Design review of the part built by this model. Coordinates are the model's own, in mm. Face numbers are marked on the shaded views. A direction names the side the tool comes from. Coordinates: 2 decimals unless noted, no trailing zeros. Write each loop counter-clockwise with the first axis right and the second up, starting at its lowest first coordinate (ties: lowest second). Pieces come first, ordered by that corner, then holes. Notation, with made-up numbers: (1, 81) -> (5, 81) arc R18 cw to (5, 94) -> close; hole circle Ø3 at (31.5, 79.25). An arc over 180 degrees is marked (long way). One line per question, with ' | ' between items. Start each with the question number.
Q1. Wall thickness on probe 1 along Y at (x, z) = (0, 8.25); probe 2 along Z at (x, y) = (13.5, 1.25); probe 3 along Z at (x, y) = (3, -7.5): over which ranges is each line inside the solid? List them lowest first.
Q2. Add section D-D on z = 8.75. State the section outline as (x, y) points, and give its area (3 significant figures).
Q3. Add section B-B on z = 0.5. State the section outline as (x, y) points, and give its area (3 significant figures).
Q4. Add section A-A on y = 0. State the section outline as (x, z) points.
Q5. Add section C-C on x = -19.5. State the section outline as (y, z) points, and give its area (3 significant figures).
Q6. For the marked faces 1 and 2, list the 3-axis set-ups (+Z, -Z, +X, -X, +Y, -Y) from which the entire face can be reached by the end or side of a thin tool; tool diameter is ignored.
Q7. For P1, Ø1, axis at x = 14, y = 5.5, coming from the +Z side; P2, Ø4, axis at x = -18.5, y = 0, coming from the +Z side; P3, Ø4, axis at x = 7, y = -4.5, coming from the +Z side; P4, Ø2, axis at y = -8, z = 6.5, coming from the +X side, all flat-tipped, find the tip position at first contact; note any pin that passes through.
Q8. Draft analysis for pull direction X (two halves, no side actions). For the marked faces 3, 4 and 5, state which applies: pulls with the +X half, pulls with the -X half, needs draft (parallel to the pull), parting line crosses it, or undercut.
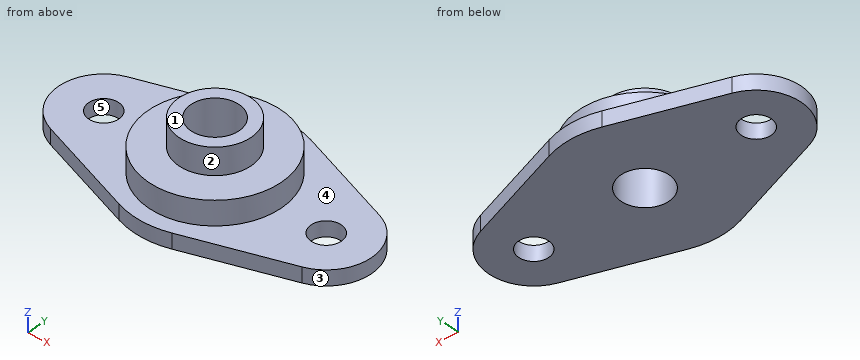
from build123d import *

# Parameters (mm, degrees)
SKETCH2_R           = 4
SKETCH2_R_2         = 2.5
BOSS_EXTRUDE1_DEPTH = 2.5
SKETCH3_R           = 6
SKETCH3_R_2         = 4
BOSS_EXTRUDE2_DEPTH = 10.922
SKETCH4_R           = 11
SKETCH4_R_2         = 6
BOSS_EXTRUDE3_DEPTH = 4


with BuildPart() as part:
    # Sketch2 → Boss-Extrude1 (new body)
    with BuildSketch(Plane.XY):
        with BuildLine():
            ThreePointArc((20.932432432, -7.094594595), (26, 0), (20.932432432, 7.094594595))
            Line((20.932432432, 7.094594595), (4.378378378, 12.77027027))
            ThreePointArc((4.378378378, 12.77027027), (0, 13.5), (-4.378378378, 12.77027027))
            Line((-4.378378378, 12.77027027), (-20.932432432, 7.094594595))
            ThreePointArc((-20.932432432, 7.094594595), (-26, 0), (-20.932432432, -7.094594595))
            Line((-20.932432432, -7.094594595), (-4.378378378, -12.77027027))
            ThreePointArc((-4.378378378, -12.77027027), (0, -13.5), (4.378378378, -12.77027027))
            Line((4.378378378, -12.77027027), (20.932432432, -7.094594595))
        make_face()
        Circle(SKETCH2_R, mode=Mode.SUBTRACT)
        with Locations((18.5, 0)):
            Circle(SKETCH2_R_2, mode=Mode.SUBTRACT)
        with Locations((-18.5, 0)):
            Circle(SKETCH2_R_2, mode=Mode.SUBTRACT)
    extrude(amount=BOSS_EXTRUDE1_DEPTH)

    # Sketch3 → Boss-Extrude2 (add)
    with BuildSketch(Plane.XY):
        Circle(SKETCH3_R)
        Circle(SKETCH3_R_2, mode=Mode.SUBTRACT)
    extrude(amount=BOSS_EXTRUDE2_DEPTH)

    # Sketch4 → Boss-Extrude3 (add)
    with BuildSketch(Plane.XY.offset(2.5)):
        Circle(SKETCH4_R)
        Circle(SKETCH4_R_2, mode=Mode.SUBTRACT)
    extrude(amount=BOSS_EXTRUDE3_DEPTH)


solid = part.part
Output values:
1) probe 1: y = -6 to -4, 4 to 6 | probe 2: z = 0 to 2.5 | probe 3: z = 0 to 6.5
2) outline: circle Ø12 at (0, 0); hole circle Ø8 at (0, 0) | area: 62.8 mm2
3) outline: (-20.93, -7.09) -> (-4.38, -12.77) arc R13.5 ccw to (4.38, -12.77) -> (20.93, -7.09) arc R7.5 ccw to (20.93, 7.09) -> (4.38, 12.77) arc R13.5 ccw to (-4.38, 12.77) -> (-20.93, 7.09) arc R7.5 ccw to start; hole circle Ø5 at (-18.5, 0); hole circle Ø8 at (0, 0); hole circle Ø5 at (18.5, 0) | area: 905 mm2
4) outline: (-26, 0) -> (-21, 0) -> (-21, 2.5) -> (-26, 2.5) -> close; (-16, 0) -> (-4, 0) -> (-4, 10.92) -> (-6, 10.92) -> (-6, 6.5) -> (-11, 6.5) -> (-11, 2.5) -> (-16, 2.5) -> close; (4, 0) -> (16, 0) -> (16, 2.5) -> (11, 2.5) -> (11, 6.5) -> (6, 6.5) -> (6, 10.92) -> (4, 10.92) -> close; (21, 0) -> (26, 0) -> (26, 2.5) -> (21, 2.5) -> close
5) outline: (-7.59, 0) -> (-2.29, 0) -> (-2.29, 2.5) -> (-7.59, 2.5) -> close; (2.29, 0) -> (7.59, 0) -> (7.59, 2.5) -> (2.29, 2.5) -> close | area: 26.5 mm2
6) face 1: +Z, +X, -X, +Y, -Y | face 2: +Z
7) P1: stops at z = 2.5 | P2: passes through | P3: stops at z = 6.5 | P4: stops at x = 8.49
8) face 3: pulls with the +X half | face 4: needs draft | face 5: undercut
